Could you check a few things on this model? Use its own coordinates, in mm. Give positions to 0.01 mm unless a question says otherwise; leave off trailing zeros. Loops run counter-clockwise (first coordinate to the right, second up) from the corner with the lowest first, then second, coordinate; pieces in that order, holes last. Notation, with made-up numbers: (-8.75, 87) - (41.25, 87) arc R27 cw to (41.25, 123) - close; hole circle Ø10 at (60, 4.25). An arc over 180 degrees is marked (long way). Write each question's results on one line, items separated by ' | '. Start each with the question number.
1) I want a section at B-B, the plane y = 0. Write out the boundary of the cut face in (x, z).
2) If we mould it in two halves opening along X, with no side actions, what happens to faces 1 (the face through (12, 0, 0)), 2 (the face through (16.5, -0.2, -0.1)), 3 (the face through (0, 1.35, 0)), 4 (the face through (-15, 0, 0))? For each: +X half, -X half, draft (parallel to the pull), parting line (faces both ways), or undercut.
3) If I drill on probe 1 along X at (y, z) = (-0.7, 0); probe 2 along Z at (x, y) = (-13.5, 0.3); probe 3 along X at (y, z) = (-0.85, 0.55), over which ranges is the centre line in solid material (lowest first)? Write a range as [from, to].
4) I want a section at A-A, the plane z = 0. Write out the boundary of the cut face in (x, y).
5) I'm going to push flat-ended pins straight in: pin 1 (1.8 mm diameter, centred on x = 13.5, z = 0, fed in from +Y); pin 2 (1.5 mm diameter, centred on y = -0.5, z = 1.5, fed in from +X). Where does each tip first touch, or does it pass through?
from build123d import *

# Parameters (mm, degrees)
SKETCH1_R           = 1.5
BOSS_EXTRUDE1_DEPTH = 1.35
CHAMFER1_SIZE       = 0.4


with BuildPart() as part:
    # Sketch1 → Boss-Extrude1 (new body, symmetric)
    with BuildSketch(Plane(origin=(0, 0, 0), x_dir=(1, 0, 0), z_dir=(0, 1, 0))):
        with BuildLine():
            Line((-13.5, 3), (13.5, 3))
            ThreePointArc((13.5, 3), (16.5, 0), (13.5, -3))
            Line((13.5, -3), (-13.5, -3))
            ThreePointArc((-13.5, -3), (-16.5, 0), (-13.5, 3))
        make_face()
        with Locations((-13.5, 0)):
            Circle(SKETCH1_R, mode=Mode.SUBTRACT)
        with Locations((13.5, 0)):
            Circle(SKETCH1_R, mode=Mode.SUBTRACT)
    extrude(amount=BOSS_EXTRUDE1_DEPTH, both=True)

    # Chamfer1
    chamfer1_edges = [part.edges().sort_by_distance(p)[0] for p in [
        (16.5, 1.35, 0),
        (0, 1.35, -3),
        (-16.5, 1.35, 0),
        (0, 1.35, 3),
    ]]
    chamfer(chamfer1_edges, length=CHAMFER1_SIZE)


solid = part.part
Answers:
1) outline: (-13.5, -3) - (13.5, -3) arc R3 ccw to (13.5, 3) - (-13.5, 3) arc R3 ccw to start; hole circle Ø3 at (-13.5, 0); hole circle Ø3 at (13.5, 0)
2) face 1: undercut | face 2: +X half | face 3: draft | face 4: undercut
3) probe 1: x = [-16.5, -15], [-12, 12], [15, 16.5] | probe 2: z = [-3, -1.5], [1.5, 3] | probe 3: x = [-16.45, -14.9], [-12.1, 12.1], [14.9, 16.45]
4) outline: (-16.5, -1.35) - (-15, -1.35) - (-15, 1.35) - (-16.1, 1.35) - (-16.5, 0.95) - close; (-12, -1.35) - (12, -1.35) - (12, 1.35) - (-12, 1.35) - close; (15, -1.35) - (16.5, -1.35) - (16.5, 0.95) - (16.1, 1.35) - (15, 1.35) - close
5) pin 1: passes through | pin 2: stops at x = 16.4
